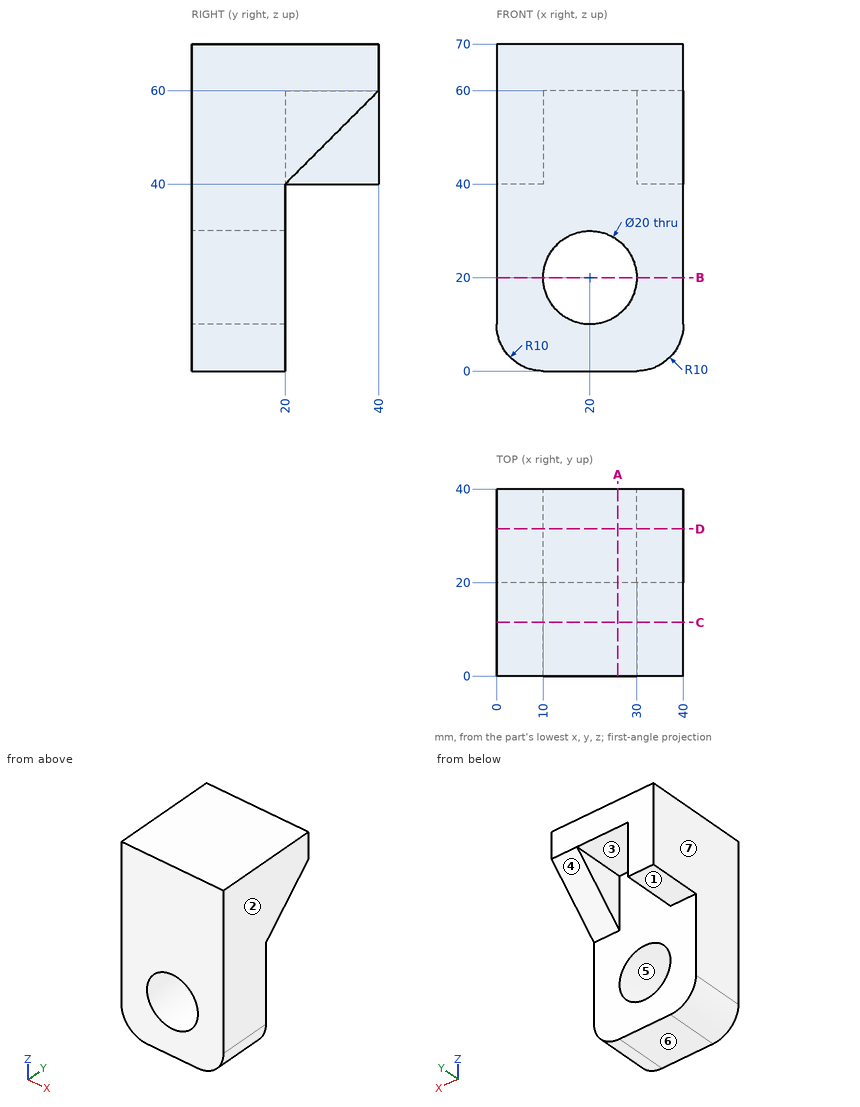
Geometry: see drawing. Coordinates: mm, zero at the bounding-box minimum. A direction names the side the tool comes from. Coordinates: 2 decimals unless noted, no trailing zeros. Loops run counter-clockwise (first coordinate to the right, second up) from the corner with the lowest first, then second, coordinate; pieces in that order, holes last. Notation, with made-up numbers: (-25, 67) - (10, 67) arc R29 cw to (10, 102) - close; hole circle Ø3 at (-36, 64.5). An arc over 180 degrees is marked (long way). Return JSON: item names as keys, results as strings.
Q1. Contact query for flat-ended pins moving along their axis: P1, Ø1.5, axis at y = 16.5, z = 7.5, coming from the -X side; P2, Ø8, axis at x = 27, z = 29.5, coming from the +Y side; P3, Ø6, axis at x = 34, y = 8.5, coming from the -Z side. Output: stop coordinate, or through.
Results:
{"P1": "x = 0.15", "P2": "y = 20", "P3": "z = 0.05"}
Q2. Section D-D, the plane y = 31.5. Return loops of the section in (x, z).
Results:
{"outline": "(0, 40) - (10, 40) - (10, 60) - (30, 60) - (30, 51.5) - (40, 51.5) - (40, 70) - (0, 70) - close"}
Q3. Section C-C, the plane y = 11.5. Return loops of the section in (x, z).
Results:
{"outline": "(0, 10) arc R10 ccw to (10, 0) - (30, 0) arc R10 ccw to (40, 10) - (40, 70) - (0, 70) - close; hole circle Ø20 at (20, 20)"}
Q4. Mould query, pull axis Z, two halves, no side actions, for the marked faces 5, 6 and 7. Classes: released by +Z, released by -Z, zero draft, split by the parting line, or undercut.
Results:
{"face 5": "undercut", "face 6": "released by -Z", "face 7": "zero draft"}
Q5. Access query for the marked faces 1, 2, 3 and 4. Directions: +Z, -Z, +X, -X, +Y, -Y. A direction counts if a zero-diameter tool reaches every point of the face in a straight line with its end or side. Return the directions, or none.
Results:
{"face 1": "-Z, +X, -X, +Y", "face 2": "+Z, -Z, +X, +Y, -Y", "face 3": "-Z, +Y", "face 4": "-Z, +X, +Y"}
Q6. Section B-B, the plane z = 20. Return loops of the section in (x, y).
Results:
{"outline": "(0, 0) - (10, 0) - (10, 20) - (0, 20) - close; (30, 0) - (40, 0) - (40, 20) - (30, 20) - close"}
Q7. Section A-A, the plane x = 26. Return loops of the section in (y, z).
Results:
{"outline": "(0, 0) - (20, 0) - (20, 12) - (0, 12) - close; (0, 28) - (20, 28) - (20, 60) - (40, 60) - (40, 70) - (0, 70) - close"}
Q8. Material intervals for line 1 along Z through (x, y) = (20, 6.25); line 2 along Y through (x, z) = (10, 32.5); line 3 along X through (y, z) = (11, 17.5), sorted ascending.
Results:
{"line 1": "0 to 10, 30 to 70", "line 2": "0 to 20", "line 3": "0 to 10.32, 29.68 to 40"}
